Autodesk Inventor part; units mm, degrees
ref_plane "YZ Plane" through (0, 0, 0) normal (1, 0, 0) x (0, 1, 0)
ref_plane "XZ Plane" through (0, 0, 0) normal (0, 1, 0) x (-1, 0, 0)
ref_plane "XY Plane" through (0, 0, 0) normal (0, 0, 1) x (1, 0, 0)
sketch "Sketch1" plane through (0, 0, 0) normal (0, 1, 0) x (-1, 0, 0)
  circle A0 centre (0, 0) radius 3.5 construction
  circle A1 centre (0, 0) radius 5
  circle A2 centre (0, 0) radius 7.5
  dimension "d0" = 7
  dimension "d1" = 10
  dimension "d2" = 15
extrude "Extrusion1" add sketch "Sketch1" against normal blind 10
sketch "Sketch2" plane through (0, -10, 0) normal (0, -1, 0) x (1, 0, 0)
  circle A0 centre (0, 0) radius 7.5
extrude "Extrusion2" add sketch "Sketch2" along normal blind 30
ref_plane "Work Plane2" through (0, -25, 0) normal (0, -1, 0) x (1, 0, 0)
mirror "Mirror1" about plane through (0, -25, 0) normal (0, -1, 0) of "Extrusion1"
properties part number "PataPolimero"
Part model, mm, in its own coordinate system. A direction names the side the tool comes from. Give positions to 0.01 mm unless a question says otherwise; leave off trailing zeros. Write each loop counter-clockwise with the first axis right and the second up, starting at its lowest first coordinate (ties: lowest second). Pieces come first, ordered by that corner, then holes.
1) Probe L1, parallel to Z at x = 0, y = -47; L2, parallel to Y at x = -0.5, z = 0.25; L3, parallel to Z at x = -0.75, y = -8.5. List the from-to ranges inside material, lowest first.
Resolved:
L1: z = -7.5 to -5, 5 to 7.5
L2: y = -40 to -10
L3: z = -7.46 to -4.94, 4.94 to 7.46
2) Pin check, flat tips, straight feed: pin 1 (5 mm diameter, centred on x = 1, z = 1.5, fed in from -Y); pin 2 (3 mm diameter, centred on x = -1, z = -2, fed in from +Y); pin 3 (2 mm diameter, centred on x = 5, y = -35.5, fed in from -Z). Stop position of each tip, or through.
Resolved:
pin 1: stops at y = -40
pin 2: stops at y = -10
pin 3: stops at z = -6.34
3) Cut at A-A on z = 0. Write the cut outline in (x, y).
Resolved:
outline: (-7.5, -50) - (-5, -50) - (-5, -40) - (5, -40) - (5, -50) - (7.5, -50) - (7.5, 0) - (5, 0) - (5, -10) - (-5, -10) - (-5, 0) - (-7.5, 0) - close
4) Cut at C-C on x = 0. Write the cut outline in (y, z).
Resolved:
outline: (-50, -7.5) - (0, -7.5) - (0, -5) - (-10, -5) - (-10, 5) - (0, 5) - (0, 7.5) - (-50, 7.5) - (-50, 5) - (-40, 5) - (-40, -5) - (-50, -5) - close
5) Cut at D-D on y = -16.5. Write the cut outline in (x, z).
Resolved:
outline: circle Ø15 at (0, 0)
6) Cut at B-B on y = -6.5. Write the cut outline in (x, z), then the cut area to 3 significant figures.
Resolved:
outline: circle Ø15 at (0, 0); hole circle Ø10 at (0, 0)
area: 98.2 mm2
7) Which spindle directions (+Z, -Z, +X, -X, +Y, -Y) get a long thin tool onto all of the face, cutting with end or side? Do faces 1 (the face through (1.08, -45.07, 4.88)), 2 (the face through (0, -10, 0)), 3 (the face through (2, -50, -5)). Say none if no direction does.
Resolved:
face 1: -Y
face 2: +Y
face 3: +Z, -Z, +X, -X, -Y
8) Two-plate mould, pull along Z, no slides. Class faces 4 (the face through (0, -40, 0)), 5 (the face through (-2, 0, -5)): released by +Z, released by -Z, zero draft, split by the parting line, or undercut.
Resolved:
face 4: undercut
face 5: zero draft
